Input: part model. Units: mm. Frame: model coordinates. A direction names the side the tool comes from. Coordinates: 2 decimals unless noted, no trailing zeros. Order: outer loops, then holes, each group sorted by start corner. A loop starts at its lowest first (then second) coordinate and runs counter-clockwise, first axis right, second up.
from build123d import *

# Parameters (mm, degrees)
SKETCH1_W           = 31.75
SKETCH1_H           = 76.2
BOSS_EXTRUDE1_DEPTH = 6.35
SKETCH2_R           = 3.81
CUT_EXTRUDE1_DEPTH  = 7.35
SKETCH3_W           = 31.75
SKETCH3_H           = 38.1
BOSS_EXTRUDE2_DEPTH = 19.05
SKETCH4_W           = 12.7
SKETCH4_H           = 38.1
CUT_EXTRUDE2_DEPTH  = 19.05
SKETCH5_W           = 12.7
SKETCH5_H           = 28.575
CUT_EXTRUDE3_DEPTH  = 7.35
SKETCH6_W           = 12.7
SKETCH6_H           = 3.81
BOSS_EXTRUDE3_DEPTH = 11.43
BOSS_EXTRUDE4_REACH = 24.225


with BuildPart() as part:
    # Sketch1 → Boss-Extrude1 (new body)
    with BuildSketch(Plane(origin=(0, 0, 0), x_dir=(1, 0, 0), z_dir=(0, 1, 0))):
        Rectangle(SKETCH1_W, SKETCH1_H)
    extrude(amount=BOSS_EXTRUDE1_DEPTH)

    # Sketch2 → Cut-Extrude1 (cut, through all)
    with BuildSketch(Plane(origin=(0, 6.35, 0), x_dir=(1, 0, 0), z_dir=(0, 1, 0))):
        with Locations((0, 25.4)):
            Circle(SKETCH2_R)
    extrude(amount=-CUT_EXTRUDE1_DEPTH, mode=Mode.SUBTRACT)

    # Sketch3 → Boss-Extrude2 (add)
    with BuildSketch(Plane(origin=(0, 6.35, 0), x_dir=(1, 0, 0), z_dir=(0, 1, 0))):
        with Locations((0, -19.05)):
            Rectangle(SKETCH3_W, SKETCH3_H)
    extrude(amount=BOSS_EXTRUDE2_DEPTH)

    # Sketch4 → Cut-Extrude2 (cut)
    with BuildSketch(Plane(origin=(0, 25.4, 0), x_dir=(1, 0, 0), z_dir=(0, 1, 0))):
        with Locations((0, -19.05)):
            Rectangle(SKETCH4_W, SKETCH4_H)
    extrude(amount=-CUT_EXTRUDE2_DEPTH, mode=Mode.SUBTRACT)

    # Sketch5 → Cut-Extrude3 (cut, through all)
    with BuildSketch(Plane(origin=(0, 6.35, 0), x_dir=(1, 0, 0), z_dir=(0, 1, 0))):
        with Locations((0, -18.0975)):
            Rectangle(SKETCH5_W, SKETCH5_H)
    extrude(amount=-CUT_EXTRUDE3_DEPTH, mode=Mode.SUBTRACT)

    # Sketch6 → Boss-Extrude3 (add)
    with BuildSketch(Plane(origin=(0, 6.35, 0), x_dir=(1, 0, 0), z_dir=(0, 1, 0))):
        with Locations((0, -1.905)):
            Rectangle(SKETCH6_W, SKETCH6_H)
    extrude(amount=BOSS_EXTRUDE3_DEPTH)

    # Sketch7 → Boss-Extrude4 (add, up to next)
    with BuildSketch(Plane(origin=(-6.35, 0, 0), x_dir=(0, 0, -1), z_dir=(1, 0, 0)), mode=Mode.PRIVATE) as boss_extrude4_sk1:
        Polygon((-32.385, 17.78), (-27.305, 17.78), (-27.305, 11.43), (-32.385, 11.43), (-32.385, 6.35), (-38.1, 6.35), (-38.1, 25.4), (-32.385, 25.4), align=None)
    boss_extrude4_tool1 = extrude(boss_extrude4_sk1.sketch, amount=BOSS_EXTRUDE4_REACH, mode=Mode.PRIVATE) - part.part
    add(boss_extrude4_tool1.solids().sort_by_distance((-6.35, 15.584714, 34.008786))[0])


solid = part.part
Item 1: Cut plane B-B on x = 0. Return loops of the section in (y, z) (3 decimals).
Response values:
outline: (0, -38.1) - (6.35, -38.1) - (6.35, -29.21) - (0, -29.21) - close; (0, -21.59) - (6.35, -21.59) - (6.35, 0) - (17.78, 0) - (17.78, 3.81) - (0, 3.81) - close; (0, 32.385) - (11.43, 32.385) - (11.43, 27.305) - (17.78, 27.305) - (17.78, 32.385) - (25.4, 32.385) - (25.4, 38.1) - (0, 38.1) - close
Item 2: Cut plane D-D on x = 11. Return loops of the section in (y, z), then the cut area to 3 significant figures.
Response values:
outline: (0, -38.1) - (6.35, -38.1) - (6.35, 0) - (25.4, 0) - (25.4, 38.1) - (0, 38.1) - close
area: 1,210 mm2
Item 3: Cut plane C-C on y = 12.75. Return loops of the section in (x, z) (3 decimals), then the cut area to 3 significant figures.
Response values:
outline: (-15.875, 0) - (15.875, 0) - (15.875, 38.1) - (-15.875, 38.1) - close; hole (-6.35, 3.81) - (6.35, 3.81) - (6.35, 27.305) - (-6.35, 27.305) - close
area: 911 mm2
Item 4: Pin query (flat end, axial travel): pin 1 Ø5 at (x, z) = (-0.5, -15.5) entering from -Y; pin 2 Ø4 at (x, y) = (-1, 22) entering from -Z (3 decimals); pin 3 Ø4 at (x, z) = (1.5, 29.5) entering from +Y; pin 4 Ø3 at (x, y) = (-1, 14.5) entering from -Z. Return the tip coordinate at first contact, or that it passes through.
Response values:
pin 1: stops at y = 0
pin 2: stops at z = 32.385
pin 3: stops at y = 17.78
pin 4: stops at z = 0
Item 5: Access query for faces 4 (the face through (0, 22, 32.385)), 5 (the face through (0, 16, 0)), 6 (the face through (15.875, 10, 9)), 7 (the face through (0, 6, 32.385)), 8 (the face through (0, 15, 27.305)). Directions: +Z, -Z, +X, -X, +Y, -Y. A direction counts if a zero-diameter tool reaches every point of the face in a straight line with its end or side. Return the directions, or none.
Response values:
face 4: -Z, +Y
face 5: -Z, +X, -X, +Y
face 6: +Z, -Z, +X, +Y, -Y
face 7: -Y
face 8: +Y, -Y
Item 6: Ray query, probe 1 along Z at (x, y) = (0, 4) (3 decimals); probe 2 along X at (y, z) = (3.25, -25.4) (3 decimals); probe 3 along Z at (x, y) = (-4.5, 15.5) (3 decimals). Return the intervals inside material, ascending.
Response values:
probe 1: z = -38.1 to -29.21, -21.59 to 3.81, 32.385 to 38.1
probe 2: x = -15.875 to -3.81, 3.81 to 15.875
probe 3: z = 0 to 3.81, 27.305 to 38.1
Item 7: Draft query along X for faces 1 (the face through (-0.83, 3.22, -21.68)), 2 (the face through (-15.875, 10, 9)), 3 (the face through (7, 25.4, 19)). Return one class per face: pulls with the +X half, pulls with the -X half, needs draft (parallel to the pull), parting line crosses it, or undercut.
Response values:
face 1: undercut
face 2: pulls with the -X half
face 3: needs draft
Item 8: Cut plane A-A on z = 16.5. Return loops of the section in (x, y) (3 decimals).
Response values:
outline: (-15.875, 0) - (-6.35, 0) - (-6.35, 25.4) - (-15.875, 25.4) - close; (6.35, 0) - (15.875, 0) - (15.875, 25.4) - (6.35, 25.4) - close
